The listing builds one solid part. Answer for the finished solid, in the listing's coordinates (mm). Face numbers are marked on the shaded views. A direction names the side the tool comes from. Round coordinates to 2 decimals unless told otherwise and drop trailing zeros. Write each loop counter-clockwise with the first axis right and the second up, starting at its lowest first coordinate (ties: lowest second). Pieces come first, ordered by that corner, then holes.
Item 1: Find the intervals of material crossed by probe 1 along X at (y, z) = (0.85, -7); probe 2 along Z at (x, y) = (-7.5, 1.25); probe 3 along X at (y, z) = (1.55, -7) (3 decimals), in increasing order.
Item 2: Find section A-A on z = -3. Give the vertices of the cut face in (x, y) (3 decimals), then the cut area to 3 significant figures.
Item 3: Find section B-B on y = 2.5. Give the vertices of the cut face in (x, z) (3 decimals).
Item 4: Find section C-C on y = 0.3. Give the vertices of the cut face in (x, z), then the cut area to 3 significant figures.
Item 5: Each of these flat-tipped pins is pushed along its axis until it touches: pin 1 (1.2 mm diameter, centred on x = 1, y = 2, fed in from +Z); pin 2 (0.6 mm diameter, centred on y = 2.5, z = -9.5, fed in from -X); pin 3 (0.9 mm diameter, centred on x = 7.5, z = -5, fed in from +Y). Where does it stop, or does it pass through?
Item 6: Find section D-D on x = 0.75. Give the vertices of the cut face in (y, z), then the cut area to 3 significant figures.
Item 7: For a pull along Z with two mould halves and no side action, classify the marked faces 6, 7, 8 and 9 as +Z half, -Z half, draft (parallel to the pull), parting line (faces both ways), or undercut.
Item 8: A tool of negligible diameter and unlimited length cuts with its end or side. For the marked faces 1, 2, 3, 4 and 5, from which of +Z, -Z, +X, -X, +Y, -Y can it reach the whole face along a straight path? Write none if from no direction.
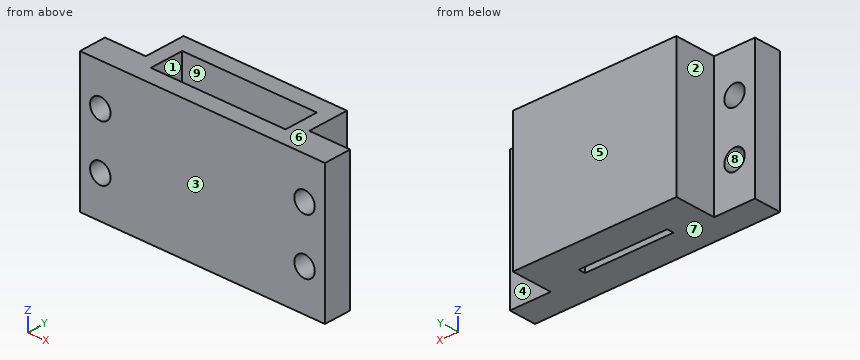
```python
from build123d import *

# Parameters (mm, degrees)
SKETCH2_W           = 6
SKETCH2_H           = 10
BOSS_EXTRUDE2_DEPTH = 5
SKETCH4_W           = 4.945
SKETCH4_H           = 2.5
CUT_EXTRUDE1_DEPTH  = 8
SKETCH6_W           = 3.25
SKETCH6_H           = 0.5
CUT_EXTRUDE2_DEPTH  = 8
SKETCH7_W           = 10
SKETCH7_H           = 1.999993684
BOSS_EXTRUDE3_DEPTH = 3
SKETCH8_W           = 10
SKETCH8_H           = 2
BOSS_EXTRUDE4_DEPTH = 3
SKETCH11_R          = 0.75
CUT_EXTRUDE7_DEPTH  = 3


with BuildPart() as part:
    # Sketch2 → Boss-Extrude2 (new body)
    with BuildSketch(Plane(origin=(0, 0, 0), x_dir=(1, 0, 0), z_dir=(0, 1, 0))):
        with Locations((-3, 5)):
            Rectangle(SKETCH2_W, SKETCH2_H)
        with Locations((3, 5)):
            Rectangle(SKETCH2_W, SKETCH2_H)
    extrude(amount=BOSS_EXTRUDE2_DEPTH)

    # Sketch4 → Cut-Extrude1 (cut)
    with BuildSketch(Plane.XY):
        with Locations((-2.4725, 2.5)):
            Rectangle(SKETCH4_W, SKETCH4_H)
        with Locations((2.4725, 2.5)):
            Rectangle(SKETCH4_W, SKETCH4_H)
    extrude(amount=-CUT_EXTRUDE1_DEPTH, mode=Mode.SUBTRACT)

    # Sketch6 → Cut-Extrude2 (cut)
    with BuildSketch(Plane(origin=(0, 0, -10), x_dir=(-1, 0, 0), z_dir=(0, 0, -1))):
        with Locations((-1.625, 2.5)):
            Rectangle(SKETCH6_W, SKETCH6_H)
        with Locations((1.625, 2.5)):
            Rectangle(SKETCH6_W, SKETCH6_H)
    extrude(amount=-CUT_EXTRUDE2_DEPTH, mode=Mode.SUBTRACT)

    # Sketch7 → Boss-Extrude3 (add)
    with BuildSketch(Plane.ZY.offset(6)):
        with Locations((-5, 0.999996842)):
            Rectangle(SKETCH7_W, SKETCH7_H)
    extrude(amount=BOSS_EXTRUDE3_DEPTH)

    # Sketch8 → Boss-Extrude4 (add)
    with BuildSketch(Plane(origin=(6, 0, 0), x_dir=(0, 0, -1), z_dir=(1, 0, 0))):
        with Locations((5, 1)):
            Rectangle(SKETCH8_W, SKETCH8_H)
    extrude(amount=BOSS_EXTRUDE4_DEPTH)

    # Sketch11 → Cut-Extrude7 (cut)
    with BuildSketch(Plane(origin=(0, 2, 0), x_dir=(1, 0, 0), z_dir=(0, 1, 0))):
        with Locations((-7.5, 7)):
            Circle(SKETCH11_R)
        with Locations((-7.5, 3)):
            Circle(SKETCH11_R)
        with Locations((7.5, 3)):
            Circle(SKETCH11_R)
        with Locations((7.5, 7)):
            Circle(SKETCH11_R)
    extrude(amount=-CUT_EXTRUDE7_DEPTH, mode=Mode.SUBTRACT)


solid = part.part
```
Check values:
1. probe 1: x = -9 to -8.25, -6.75 to 6.75, 8.25 to 9
1. probe 2: z = -10 to -7.75, -6.25 to -3.75, -2.25 to 0
1. probe 3: x = -9 to -8.25, -6.75 to -4.945, 4.945 to 6.75, 8.25 to 9
2. outline: (-9, 0) - (-8.25, 0) - (-8.25, 2) - (-9, 2) - close; (-6.75, 0) - (6.75, 0) - (6.75, 2) - (6, 2) - (6, 5) - (-6, 5) - (-6, 2) - (-6.75, 2) - close; (8.25, 0) - (9, 0) - (9, 2) - (8.25, 2) - close; hole (-4.945, 1.25) - (4.945, 1.25) - (4.945, 3.75) - (-4.945, 3.75) - close
2. area: 41.3 mm2
3. outline: (-6, -10) - (-3.25, -10) - (-3.25, -8) - (-4.945, -8) - (-4.945, 0) - (-6, 0) - close; (3.25, -10) - (6, -10) - (6, 0) - (4.945, 0) - (4.945, -8) - (3.25, -8) - close
4. outline: (-9, -10) - (9, -10) - (9, 0) - (-9, 0) - close; hole circle Ø1.5 at (-7.5, -7); hole circle Ø1.5 at (-7.5, -3); hole circle Ø1.5 at (7.5, -7); hole circle Ø1.5 at (7.5, -3)
4. area: 173 mm2
5. pin 1: stops at z = -8
5. pin 2: stops at x = -6
5. pin 3: stops at y = 2
6. outline: (0, -10) - (2.25, -10) - (2.25, -8) - (1.25, -8) - (1.25, 0) - (0, 0) - close; (2.75, -10) - (5, -10) - (5, 0) - (3.75, 0) - (3.75, -8) - (2.75, -8) - close
6. area: 29.0 mm2
7. face 6: +Z half
7. face 7: -Z half
7. face 8: undercut
7. face 9: draft
8. face 1: +Z
8. face 2: +Z, -Z, -X, +Y
8. face 3: +Z, -Z, +X, -X, -Y
8. face 4: +Z, -Z, +X, +Y
8. face 5: +Z, -Z, +X, -X, +Y
